Part model, mm, in its own coordinate system. A direction names the side the tool comes from. Round coordinates to 2 decimals unless told otherwise and drop trailing zeros. Write each loop counter-clockwise with the first axis right and the second up, starting at its lowest first coordinate (ties: lowest second). Pieces come first, ordered by that corner, then holes. Notation, with made-up numbers: M 7,71.25 L 25,71.25 A32 ccw 25,101.25 Z; hole C -34.75,18 d6. An arc over 180 degrees is marked long. Use one line per item in the form item = value. Start each with the question number.
Item 1: Which spindle directions (+Z, -Z, +X, -X, +Y, -Y) get a long thin tool onto all of the face, cutting with end or side? Do faces 5 (the face through (16.91, 10.11, -23.98)), 6 (the face through (18.93, 10.11, 7.87)), 7 (the face through (-23.98, 10.11, -16.91)). Say none if no direction does.
Item 2: Cut at A-A, the plane x = 0. Give the cut face in (y, z), then the cut area to 4 significant figures.
Item 3: Cut at D-D, the plane z = -34. Give the cut face in (x, y), then the cut area to 3 significant figures.
Item 4: Probe L1, parallel to Z at x = -26.5, y = 4; L2, parallel to X at y = 11.5, z = -34.5. List the from-to ranges inside material, lowest first.
Item 5: Cut at B-B, the plane z = 0. Give the cut face in (x, y).
Item 6: Mould opens along X. For faces 1 (the face through (4.2, 10.106, -38.986)), 2 (the face through (29, 10, -5)), 3 (the face through (-5, 10, -29)), 4 (the face through (-28.26, 10.11, -28.31)) say: +X half, -X half, draft (parallel to the pull), parting line (faces both ways), or undercut.
Item 7: Cut at C-C, the plane x = -15. Give the cut face in (y, z), then the cut area to 3 significant figures.
Item 8: Flat gauge pins, fed straight in: pin 1 Ø8 at (x, y) = (-32.5, 10) entering from +Z; pin 2 Ø1.5 at (x, z) = (-17, -14.5) entering from +Y; pin 3 Ø5 at (x, y) = (-24.5, 2.5) entering from +Z. Where does each tip first touch, or does it go through?
from build123d import *

# Parameters (mm, degrees)
SKETCH1_R           = 17.5
BOSS_EXTRUDE1_DEPTH = 20.5
SKETCH2_R           = 2.5
BOSS_EXTRUDE2_DEPTH = 1
SKETCH3_R           = 2.394052793
BOSS_EXTRUDE3_DEPTH = 1


with BuildPart() as part:
    # Sketch1 → Boss-Extrude1 (new body)
    with BuildSketch(Plane(origin=(0, 0, 0), x_dir=(1, 0, 0), z_dir=(0, 1, 0))):
        with BuildLine():
            Line((5, 20.645822822), (5, 36.945906404))
            ThreePointArc((5, 36.945906404), (4.177898814, 39.00909732), (2.162162162, 39.941520437))
            ThreePointArc((2.162162162, 39.941520437), (0, 40), (-2.162162162, 39.941520437))
            ThreePointArc((-2.162162162, 39.941520437), (-4.177898814, 39.00909732), (-5, 36.945906404))
            Line((-5, 36.945906404), (-5, 20.645822822))
            ThreePointArc((-5, 20.645822822), (-5.200290751, 20.04543535), (-5.720930233, 19.685551993))
            ThreePointArc((-5.720930233, 19.685551993), (-7.845010363, 18.939530416), (-9.874478744, 17.965095868))
            ThreePointArc((-9.874478744, 17.965095868), (-10.497102414, 17.851424122), (-11.063267415, 18.134335227))
            Line((-11.063267415, 18.134335227), (-22.589167049, 29.660234861))
            ThreePointArc((-22.589167049, 29.660234861), (-24.629376661, 30.537817825), (-26.714040425, 29.771799478))
            ThreePointArc((-26.714040425, 29.771799478), (-28.284271247, 28.284271247), (-29.771799478, 26.714040425))
            ThreePointArc((-29.771799478, 26.714040425), (-30.537817825, 24.629376661), (-29.660234861, 22.589167049))
            Line((-29.660234861, 22.589167049), (-18.134335227, 11.063267415))
            ThreePointArc((-18.134335227, 11.063267415), (-17.851424122, 10.497102414), (-17.965095868, 9.874478744))
            ThreePointArc((-17.965095868, 9.874478744), (-18.939530416, 7.845010363), (-19.685551993, 5.720930233))
            ThreePointArc((-19.685551993, 5.720930233), (-20.04543535, 5.200290751), (-20.645822822, 5))
            Line((-20.645822822, 5), (-36.945906404, 5))
            ThreePointArc((-36.945906404, 5), (-39.00909732, 4.177898814), (-39.941520437, 2.162162162))
            ThreePointArc((-39.941520437, 2.162162162), (-40, 0), (-39.941520437, -2.162162162))
            ThreePointArc((-39.941520437, -2.162162162), (-39.00909732, -4.177898814), (-36.945906404, -5))
            Line((-36.945906404, -5), (-20.645822822, -5))
            ThreePointArc((-20.645822822, -5), (-20.04543535, -5.200290751), (-19.685551993, -5.720930233))
            ThreePointArc((-19.685551993, -5.720930233), (-18.939530416, -7.845010363), (-17.965095868, -9.874478744))
            ThreePointArc((-17.965095868, -9.874478744), (-17.851424122, -10.497102414), (-18.134335227, -11.063267415))
            Line((-18.134335227, -11.063267415), (-29.660234861, -22.589167049))
            ThreePointArc((-29.660234861, -22.589167049), (-30.537817825, -24.629376661), (-29.771799478, -26.714040425))
            ThreePointArc((-29.771799478, -26.714040425), (-28.284271247, -28.284271247), (-26.714040425, -29.771799478))
            ThreePointArc((-26.714040425, -29.771799478), (-24.629376661, -30.537817825), (-22.589167049, -29.660234861))
            Line((-22.589167049, -29.660234861), (-11.063267415, -18.134335227))
            ThreePointArc((-11.063267415, -18.134335227), (-10.497102414, -17.851424122), (-9.874478744, -17.965095868))
            ThreePointArc((-9.874478744, -17.965095868), (-7.845010363, -18.939530416), (-5.720930233, -19.685551993))
            ThreePointArc((-5.720930233, -19.685551993), (-5.200290751, -20.04543535), (-5, -20.645822822))
            Line((-5, -20.645822822), (-5, -36.945906404))
            ThreePointArc((-5, -36.945906404), (-4.177898814, -39.00909732), (-2.162162162, -39.941520437))
            ThreePointArc((-2.162162162, -39.941520437), (0, -40), (2.162162162, -39.941520437))
            ThreePointArc((2.162162162, -39.941520437), (4.177898814, -39.00909732), (5, -36.945906404))
            Line((5, -36.945906404), (5, -20.645822822))
            ThreePointArc((5, -20.645822822), (5.200290751, -20.04543535), (5.720930233, -19.685551993))
            ThreePointArc((5.720930233, -19.685551993), (7.845010363, -18.939530416), (9.874478744, -17.965095868))
            ThreePointArc((9.874478744, -17.965095868), (10.497102414, -17.851424122), (11.063267415, -18.134335227))
            Line((11.063267415, -18.134335227), (22.589167049, -29.660234861))
            ThreePointArc((22.589167049, -29.660234861), (24.629376661, -30.537817825), (26.714040425, -29.771799478))
            ThreePointArc((26.714040425, -29.771799478), (28.284271247, -28.284271247), (29.771799478, -26.714040425))
            ThreePointArc((29.771799478, -26.714040425), (30.537817825, -24.629376661), (29.660234861, -22.589167049))
            Line((29.660234861, -22.589167049), (18.134335227, -11.063267415))
            ThreePointArc((18.134335227, -11.063267415), (17.851424122, -10.497102414), (17.965095868, -9.874478744))
            ThreePointArc((17.965095868, -9.874478744), (18.939530416, -7.845010363), (19.685551993, -5.720930233))
            ThreePointArc((19.685551993, -5.720930233), (20.04543535, -5.200290751), (20.645822822, -5))
            Line((20.645822822, -5), (36.945906404, -5))
            ThreePointArc((36.945906404, -5), (39.00909732, -4.177898814), (39.941520437, -2.162162162))
            ThreePointArc((39.941520437, -2.162162162), (40, 0), (39.941520437, 2.162162162))
            ThreePointArc((39.941520437, 2.162162162), (39.00909732, 4.177898814), (36.945906404, 5))
            Line((36.945906404, 5), (20.645822822, 5))
            ThreePointArc((20.645822822, 5), (20.04543535, 5.200290751), (19.685551993, 5.720930233))
            ThreePointArc((19.685551993, 5.720930233), (18.939530416, 7.845010363), (17.965095868, 9.874478744))
            ThreePointArc((17.965095868, 9.874478744), (17.851424122, 10.497102414), (18.134335227, 11.063267415))
            Line((18.134335227, 11.063267415), (29.660234861, 22.589167049))
            ThreePointArc((29.660234861, 22.589167049), (30.537817825, 24.629376661), (29.771799478, 26.714040425))
            ThreePointArc((29.771799478, 26.714040425), (28.284271247, 28.284271247), (26.714040425, 29.771799478))
            ThreePointArc((26.714040425, 29.771799478), (24.629376661, 30.537817825), (22.589167049, 29.660234861))
            Line((22.589167049, 29.660234861), (11.063267415, 18.134335227))
            ThreePointArc((11.063267415, 18.134335227), (10.497102414, 17.851424122), (9.874478744, 17.965095868))
            ThreePointArc((9.874478744, 17.965095868), (7.845010363, 18.939530416), (5.720930233, 19.685551993))
            ThreePointArc((5.720930233, 19.685551993), (5.200290751, 20.04543535), (5, 20.645822822))
        make_face()
        with Locations(Location((0, 0, 0), (0, 0, 270))):
            Circle(SKETCH1_R, mode=Mode.SUBTRACT)
    extrude(amount=BOSS_EXTRUDE1_DEPTH)

    # Sketch2 → Boss-Extrude2 (add)
    with BuildSketch(Plane(origin=(0, 20.5, 0), x_dir=(1, 0, 0), z_dir=(0, 1, 0))):
        with Locations(Location((0, 30, 0), (0, 0, 270))):
            Circle(SKETCH2_R)
        with Locations(Location((30, 0, 0), (0, 0, 270))):
            Circle(SKETCH2_R)
        with Locations(Location((0, -30, 0), (0, 0, 270))):
            Circle(SKETCH2_R)
        with Locations(Location((-30, 0, 0), (0, 0, 270))):
            Circle(SKETCH2_R)
    extrude(amount=BOSS_EXTRUDE2_DEPTH)

    # Sketch3 → Boss-Extrude3 (add)
    with BuildSketch(Plane.XZ):
        with Locations(Location((-21.213203436, 21.213203436, 0), (0, 0, 90))):
            Circle(SKETCH3_R)
        with Locations(Location((21.213203436, 21.213203436, 0), (0, 0, 90))):
            Circle(SKETCH3_R)
        with Locations(Location((21.213203436, -21.213203436, 0), (0, 0, 90))):
            Circle(SKETCH3_R)
        with Locations(Location((-21.213203436, -21.213203436, 0), (0, 0, 90))):
            Circle(SKETCH3_R)
    extrude(amount=BOSS_EXTRUDE3_DEPTH)


solid = part.part
Model answer:
q1.face_5 = -Z, +Y, -Y
q1.face_6 = +X, +Y, -Y
q1.face_7 = -X, +Y, -Y
q2.outline = M 0,-40 L 20.5,-40 L 20.5,-32.5 L 21.5,-32.5 L 21.5,-27.5 L 20.5,-27.5 L 20.5,-17.5 L 0,-17.5 Z; M 0,17.5 L 20.5,17.5 L 20.5,27.5 L 21.5,27.5 L 21.5,32.5 L 20.5,32.5 L 20.5,40 L 0,40 Z
q2.area = 932.5 mm²
q3.outline = M -5,0 L 5,0 L 5,20.5 L -5,20.5 Z
q3.area = 205 mm²
q4.L1 = -29.95 to -19.43, -5 to 5, 19.43 to 29.95
q4.L2 = -5 to 5
q5.outline = M -40,0 L -17.5,0 L -17.5,20.5 L -27.5,20.5 L -27.5,21.5 L -32.5,21.5 L -32.5,20.5 L -40,20.5 Z; M 17.5,0 L 40,0 L 40,20.5 L 32.5,20.5 L 32.5,21.5 L 27.5,21.5 L 27.5,20.5 L 17.5,20.5 Z
q6.face_1 = +X half
q6.face_2 = draft
q6.face_3 = undercut
q6.face_4 = -X half
q7.outline = M 0,-22.07 L 20.5,-22.07 L 20.5,-9.01 L 0,-9.01 Z; M 0,9.01 L 20.5,9.01 L 20.5,22.07 L 0,22.07 Z
q7.area = 535 mm²
q8.pin_1 = 28.07
q8.pin_2 = 20.5
q8.pin_3 = 30.54
